The listing builds one solid part. Answer for the finished solid, in the listing's coordinates (mm). A direction names the side the tool comes from. Coordinates: 2 decimals unless noted, no trailing zeros. Order: outer loops, then holes, each group sorted by start corner. A loop starts at its lowest first (then second) coordinate and runs counter-clockwise, first axis right, second up.
```python
from build123d import *

# Parameters (mm, degrees)
F0_W         = 113
F0_H         = 32
F1_DEPTH     = 64
F2_W         = 25
F2_H         = 32
F3_DEPTH     = 53.5432
F4_W         = 35
F4_H         = 17
F5_DEPTH     = 34.544
F6_SIZE      = 10
F7_W         = 25
F7_H         = 34
F8_DEPTH     = 33.274
F9_R         = 5.5
F10_DEPTH    = 25.4
F11_R        = 6.5
F12_DEPTH    = 82.296
F13_T1_DEPTH = 101.7833830538
F13_T3_DEPTH = 101.7833830538


# Not quite as in the source:
# - a fillet or chamfer that OpenCascade refuses, or shapes differently, is made with other operations: its cross-section is extruded or revolved along the edge and cut away or added


with BuildPart() as f1:
    # F0 (on Top) → F1 (new body)
    with BuildSketch(Plane.XY):
        with Locations((-26.9756987691, -17.7779501617)):
            Rectangle(F0_W, F0_H)
    extrude(amount=F1_DEPTH)

    # F2 (on face) → F3 (cut)
    with BuildSketch(Plane.XY.offset(64)):
        with Locations((-70.9756987691, -17.7779501617)):
            Rectangle(F2_W, F2_H)
        with Locations((17.0243012309, -17.7779501617)):
            Rectangle(F2_W, F2_H)
    extrude(amount=-F3_DEPTH, mode=Mode.SUBTRACT)

    # F4 (on face) → F5 (cut)
    with BuildSketch(Plane.XZ.offset(33.7779501617)):
        with Locations((-26.9756987691, 8.5)):
            Rectangle(F4_W, F4_H)
    extrude(amount=-F5_DEPTH, mode=Mode.SUBTRACT)

    # F6
    f6_edges = [f1.edges().sort_by_distance(p)[0] for p in [
        (29.524301, -33.77795, 5.2284),
        (-83.475699, -33.77795, 5.2284),
    ]]
    chamfer(f6_edges, length=F6_SIZE)

    # F7 (on face) → F8 (cut)
    with BuildSketch(Plane.XZ.offset(33.7779501617)):
        with Locations((-26.9756987691, 47)):
            Rectangle(F7_W, F7_H)
    extrude(amount=-F8_DEPTH, mode=Mode.SUBTRACT)

    # F9 (on face) → F10 (cut)
    with BuildSketch(Plane.XY.offset(10.4568)):
        with Locations((-70.4708987691, -14.7827501617)):
            Circle(F9_R)
        with Locations((16.5243012309, -14.7779501617)):
            Circle(F9_R)
    extrude(amount=-F10_DEPTH, mode=Mode.SUBTRACT)

    # F11 (on face) → F12 (cut)
    with BuildSketch(Plane.YZ.offset(4.5243012309)):
        with Locations((-17.7779501617, 46)):
            Circle(F11_R)
    extrude(amount=-F12_DEPTH, mode=Mode.SUBTRACT)

    # F13: fillet of radius 16.5566766108 on 4 edges, made by hand

    # F13_s2 → F13_t1 (cut)
    with BuildSketch(Plane.YZ.offset(-55.867390296)):
        with BuildLine():
            add(Edge.make_bspline(
                [(-33.7779501617, 47.4433233892), (-33.7779501617, 64), (-17.2212735509, 64)],
                knots=[0, 0, 0, 1, 1, 1], degree=2, weights=[1, 1, 1]))
            Line((-17.2212735509, 64), (-33.7779501617, 64))
            Line((-33.7779501617, 64), (-33.7779501617, 47.4433233892))
        make_face()
        with BuildLine():
            add(Edge.make_bspline(
                [(-1.7779501617, 47.4433233892), (-1.7779501617, 64), (-18.3346267724, 64)],
                knots=[0, 0, 0, 1, 1, 1], degree=2, weights=[1, 1, 1]))
            Line((-18.3346267724, 64), (-1.7779501617, 64))
            Line((-1.7779501617, 64), (-1.7779501617, 47.4433233892))
        make_face()
    extrude(amount=F13_T1_DEPTH, mode=Mode.SUBTRACT)

    # F13_s4 → F13_t3 (cut)
    with BuildSketch(Plane.YZ.offset(-99.867390296)):
        with BuildLine():
            add(Edge.make_bspline(
                [(-33.7779501617, 47.4433233892), (-33.7779501617, 64), (-17.2212735509, 64)],
                knots=[0, 0, 0, 1, 1, 1], degree=2, weights=[1, 1, 1]))
            Line((-17.2212735509, 64), (-33.7779501617, 64))
            Line((-33.7779501617, 64), (-33.7779501617, 47.4433233892))
        make_face()
        with BuildLine():
            add(Edge.make_bspline(
                [(-1.7779501617, 47.4433233892), (-1.7779501617, 64), (-18.3346267724, 64)],
                knots=[0, 0, 0, 1, 1, 1], degree=2, weights=[1, 1, 1]))
            Line((-18.3346267724, 64), (-1.7779501617, 64))
            Line((-1.7779501617, 64), (-1.7779501617, 47.4433233892))
        make_face()
    extrude(amount=F13_T3_DEPTH, mode=Mode.SUBTRACT)


solid = f1.part
```
(1) Find section C-C (x = -30). Write down the section's boundary in (y, z), and give its area (3 significant figures).
(2) Find section B-B (z = 46). Write down the section's boundary in (x, y).
(3) Find section A-A (z = 13.5). Write down the section's boundary in (x, y), and give its area (3 significant figures).
(4) Each of these flat-tipped pins is pushed along its axis until it touches: pin 1 Ø6 at (x, y) = (-21.5, -7.5) entering from +Z; pin 2 Ø12.5 at (x, y) = (-73, -14.5) entering from +Z; pin 3 Ø12 at (y, z) = (-23.5, 19.5) entering from +X. Where does it stop, or does it pass through?
(5) The mould has two halves that part along Y. Classify faces 6 (the face through (-28, -1.778, 23)), 7 (the face through (12.16, -18.125, 5.302)), 8 (the face through (-28, -33.778, 18)), 9 (the face through (-48.8, -22.9, 42)): released by +Y, released by -Y, zero draft, split by the parting line, or undercut.
(6) Find section D-D (y = -22). Give the number of separate pieces and of enclosed holes in the cut face, and give its area (3 significant figures).
(7) For faces 1 (the face through (17, -21, 10.457)), 2 (the face through (-71, -21, 10.457)), 3 (the face through (-9.476, -18, 8)), 4 (the face through (-4.8, -22.9, 42)), 5 (the face through (-14.476, -18, 39)), determine the directions among +Z, -Z, +X, -X, +Y, -Y from which every point of the face is accessible in a straight line to the end or side of a thin tool.
(8) Consider line 1 (X direction, y = -8, z = 55.5); line 2 (Z direction, x = 11, y = -9); line 3 (Z direction, x = -29.5, y = -18). Determine where each line is inside the solid, lowest interval first.
Findings below:
1. outline: (-33.78, 17) - (-1.78, 17) - (-1.78, 30) - (-33.78, 30) - close
1. area: 416 mm2
2. outline: (-58.48, -33.78) - (-39.48, -33.78) - (-39.48, -24.28) - (-58.48, -24.28) - close; (-58.48, -11.28) - (-39.48, -11.28) - (-39.48, -1.78) - (-58.48, -1.78) - close; (-14.48, -33.78) - (4.52, -33.78) - (4.52, -24.28) - (-14.48, -24.28) - close; (-14.48, -11.28) - (4.52, -11.28) - (4.52, -1.78) - (-14.48, -1.78) - close
3. outline: (-58.48, -33.78) - (-44.48, -33.78) - (-44.48, -1.78) - (-58.48, -1.78) - close; (-9.48, -33.78) - (4.52, -33.78) - (4.52, -1.78) - (-9.48, -1.78) - close
3. area: 896 mm2
4. pin 1: stops at z = 30
4. pin 2: stops at z = 10.46
4. pin 3: stops at x = 4.52
5. face 6: released by +Y
5. face 7: undercut
5. face 8: released by -Y
5. face 9: undercut
6. separate pieces: 3
6. enclosed holes: 0
6. area: 2,720 mm2
7. face 1: +Z, +X, +Y, -Y
7. face 2: +Z, -X, +Y, -Y
7. face 3: -Z, +Y, -Y
7. face 4: +X, -X
7. face 5: +Z, +Y, -Y
8. line 1: x = -58.48 to -39.48, -14.48 to 4.52
8. line 2: z = 0 to 10.46
8. line 3: z = 17 to 30
